Read the model definition and answer for the solid it produces. Units are mm, in the model's axes. A direction names the side the tool comes from. Coordinates: 2 decimals unless noted, no trailing zeros. Loops run counter-clockwise (first coordinate to the right, second up) from the corner with the lowest first, then second, coordinate; pieces in that order, holes last. Notation, with made-up numbers: M 13.25,31 L 17.25,31 A8 cw 17.25,35 Z; hole C 10.25,-10.75 d3. An arc over 180 degrees is marked long. One line per item, written item: value. Start each with the question number.
```python
from build123d import *

# Parameters (mm, degrees)
SKETCH1_R            = 1.5
SKETCH1_R_2          = 2.5
BOSS_EXTRUDE1_DEPTH  = 5
M2_CLEARANCE_HOLE1_D = 2.4
FILLET1_R            = 2
BOSS_EXTRUDE2_START  = 5
BOSS_EXTRUDE2_DEPTH  = 5
CUT_EXTRUDE1_START   = -3
SKETCH5_R            = 1.5
CUT_EXTRUDE1_DEPTH   = 3
CUT_EXTRUDE2_START   = -2
SKETCH6_R            = 1.2
CUT_EXTRUDE2_DEPTH   = 2


with BuildPart() as part:
    # Sketch1 → Boss-Extrude1 (new body)
    # profile 1 of 3: a face of its own
    with BuildSketch(Plane(origin=(0, 0, 0), x_dir=(1, 0, 0), z_dir=(0, 1, 0))):
        with BuildLine():
            Line((10.5, 2.5), (-10.5, 2.5))
            ThreePointArc((-10.5, 2.5), (-8.732233047, 1.767766953), (-8, 0))
            ThreePointArc((-8, 0), (-10.997961344, -2.449904998), (-12.8016276, 0.975966388))
            Line((-12.8016276, 0.975966388), (-18.090408136, -11.496597633))
            Line((-18.090408136, -11.496597633), (-13.587005769, -16))
            Line((-13.587005769, -16), (13.587005769, -16))
            Line((13.587005769, -16), (18.090408136, -11.496597633))
            Line((18.090408136, -11.496597633), (12.8016276, 0.975966388))
            ThreePointArc((12.8016276, 0.975966388), (12.949904998, 0.497961344), (13, 0))
            ThreePointArc((13, 0), (8.732233047, -1.767766953), (10.5, 2.5))
        make_face()
        with Locations(Location((-14.4, -12.5, 0), (0, 0, 270))):
            Circle(SKETCH1_R, mode=Mode.SUBTRACT)
        with Locations(Location((14.4, -12.5, 0), (0, 0, 270))):
            Circle(SKETCH1_R, mode=Mode.SUBTRACT)
        Polygon((-7.5, -12.5), (0, -2), (7.5, -12.5), align=None, mode=Mode.SUBTRACT)
    # profile 2 of 3: a face of its own
    with BuildSketch(Plane(origin=(0, 0, 0), x_dir=(1, 0, 0), z_dir=(0, 1, 0))):
        with Locations((-10.5, 0)):
            Circle(SKETCH1_R_2)
    # profile 3 of 3: a face of its own
    with BuildSketch(Plane(origin=(0, 0, 0), x_dir=(1, 0, 0), z_dir=(0, 1, 0))):
        with Locations((10.5, 0)):
            Circle(SKETCH1_R_2)
    extrude(amount=BOSS_EXTRUDE1_DEPTH)

    # M2 Clearance Hole1 (through all)
    with Locations(Plane(origin=(0, 5, 0), x_dir=(1, 0, 0), z_dir=(0, 1, 0))):
        with Locations((-10.5, 0), (10.5, 0)):
            Hole(M2_CLEARANCE_HOLE1_D / 2)

    # Fillet1
    fillet1_edges = [part.edges().sort_by_distance(p)[0] for p in [
        (0, 2.5, 2),
        (-7.5, 2.5, 12.5),
        (7.5, 2.5, 12.5),
    ]]
    fillet(fillet1_edges, radius=FILLET1_R)

    # Sketch4 → Boss-Extrude2 (add)
    with BuildSketch(Plane.XZ.offset(BOSS_EXTRUDE2_START)):
        with BuildLine():
            Line((-14.101857368, 15.4851484), (-17.3851484, 12.201857368))
            ThreePointArc((-17.3851484, 12.201857368), (-15.317017203, 9.643589762), (-12.146233974, 10.519964975))
            ThreePointArc((-12.146233974, 10.519964975), (-12.695571974, 11.154604627), (-13.01161859, 11.932199807))
            ThreePointArc((-13.01161859, 11.932199807), (-15.9, 12.5), (-13.01161859, 13.067800193))
            ThreePointArc((-13.01161859, 13.067800193), (-12.695571974, 13.845395373), (-12.146233974, 14.480035025))
            ThreePointArc((-12.146233974, 14.480035025), (-13.028642033, 15.168216132), (-14.101857368, 15.4851484))
        make_face()
        with BuildLine():
            ThreePointArc((12.146233974, 10.519964975), (15.317017203, 9.643589762), (17.3851484, 12.201857368))
            Line((17.3851484, 12.201857368), (14.101857368, 15.4851484))
            ThreePointArc((14.101857368, 15.4851484), (13.028642033, 15.168216132), (12.146233974, 14.480035025))
            ThreePointArc((12.146233974, 14.480035025), (12.695571974, 13.845395373), (13.01161859, 13.067800193))
            ThreePointArc((13.01161859, 13.067800193), (15.9, 12.5), (13.01161859, 11.932199807))
            ThreePointArc((13.01161859, 11.932199807), (12.695571974, 11.154604627), (12.146233974, 10.519964975))
        make_face()
    extrude(amount=-BOSS_EXTRUDE2_DEPTH)

    # Sketch5 → Cut-Extrude1 (cut)
    # profile 1 of 2: a face of its own
    with BuildSketch(Plane(origin=(0, 5, 0), x_dir=(1, 0, 0), z_dir=(0, 1, 0)).offset(CUT_EXTRUDE1_START)):
        Polygon((15.109788915, -15.148968295), (17.048968295, -13.209788915), (16.33917938, -10.56082062), (13.690211085, -9.851031705), (11.751031705, -11.790211085), (12.46082062, -14.43917938), align=None)
        with Locations(Location((14.4, -12.5, 0), (0, 0, 157.757128517))):
            Circle(SKETCH5_R, mode=Mode.SUBTRACT)
    # profile 2 of 2: a face of its own
    with BuildSketch(Plane(origin=(0, 5, 0), x_dir=(1, 0, 0), z_dir=(0, 1, 0)).offset(CUT_EXTRUDE1_START)):
        Polygon((-12.46082062, -14.43917938), (-15.109788915, -15.148968295), (-17.048968295, -13.209788915), (-16.33917938, -10.56082062), (-13.690211085, -9.851031705), (-11.751031705, -11.790211085), align=None)
    extrude(amount=CUT_EXTRUDE1_DEPTH, mode=Mode.SUBTRACT)

    # Sketch6 → Cut-Extrude2 (cut)
    # profile 1 of 6: a face of its own
    with BuildSketch(Plane(origin=(0, 5, 0), x_dir=(1, 0, 0), z_dir=(0, 1, 0)).offset(CUT_EXTRUDE2_START)):
        with BuildLine():
            Line((-7.757586221, 0), (-9.128793111, 2.375))
            Line((-9.128793111, 2.375), (-11.28062475, 2.375))
            ThreePointArc((-11.28062475, 2.375), (-11.75, 2.165063509), (-12.166497959, 1.863540864))
            Line((-12.166497959, 1.863540864), (-13.140949749, 0.175740855))
            Line((-13.140949749, 0.175740855), (-13.226879096, -0.026906859))
            Line((-13.226879096, -0.026906859), (-11.871206889, -2.375))
            Line((-11.871206889, -2.375), (-9.128793111, -2.375))
            Line((-9.128793111, -2.375), (-7.757586221, 0))
        make_face()
        with Locations(Location((-10.5, 0, 0), (0, 0, 270))):
            Circle(SKETCH6_R, mode=Mode.SUBTRACT)
    # profile 2 of 6: a face of its own
    with BuildSketch(Plane(origin=(0, 5, 0), x_dir=(1, 0, 0), z_dir=(0, 1, 0)).offset(CUT_EXTRUDE2_START)):
        with BuildLine():
            Line((-13.140949749, 0.175740855), (-12.166497959, 1.863540864))
            ThreePointArc((-12.166497959, 1.863540864), (-12.533089331, 1.454835995), (-12.8016276, 0.975966388))
            Line((-12.8016276, 0.975966388), (-13.140949749, 0.175740855))
        make_face()
    # profile 3 of 6: a face of its own
    with BuildSketch(Plane(origin=(0, 5, 0), x_dir=(1, 0, 0), z_dir=(0, 1, 0)).offset(CUT_EXTRUDE2_START)):
        with BuildLine():
            Line((-9.128793111, 2.375), (-9.200961894, 2.5))
            Line((-9.200961894, 2.5), (-10.5, 2.5))
            ThreePointArc((-10.5, 2.5), (-10.895284708, 2.468552207), (-11.28062475, 2.375))
            Line((-11.28062475, 2.375), (-9.128793111, 2.375))
        make_face()
    # profile 4 of 6: a face of its own
    with BuildSketch(Plane(origin=(0, 5, 0), x_dir=(1, 0, 0), z_dir=(0, 1, 0)).offset(CUT_EXTRUDE2_START)):
        with BuildLine():
            Line((7.757586221, 0), (9.128793111, -2.375))
            Line((9.128793111, -2.375), (11.871206889, -2.375))
            Line((11.871206889, -2.375), (13.226879096, -0.026906859))
            Line((13.226879096, -0.026906859), (13.140949749, 0.175740855))
            Line((13.140949749, 0.175740855), (12.166497959, 1.863540864))
            ThreePointArc((12.166497959, 1.863540864), (11.75, 2.165063509), (11.28062475, 2.375))
            Line((11.28062475, 2.375), (9.128793111, 2.375))
            Line((9.128793111, 2.375), (7.757586221, 0))
        make_face()
        with Locations(Location((10.5, 0, 0), (0, 0, 270))):
            Circle(SKETCH6_R, mode=Mode.SUBTRACT)
    # profile 5 of 6: a face of its own
    with BuildSketch(Plane(origin=(0, 5, 0), x_dir=(1, 0, 0), z_dir=(0, 1, 0)).offset(CUT_EXTRUDE2_START)):
        with BuildLine():
            Line((12.166497959, 1.863540864), (13.140949749, 0.175740855))
            Line((13.140949749, 0.175740855), (12.8016276, 0.975966388))
            ThreePointArc((12.8016276, 0.975966388), (12.533089331, 1.454835995), (12.166497959, 1.863540864))
        make_face()
    # profile 6 of 6: a face of its own
    with BuildSketch(Plane(origin=(0, 5, 0), x_dir=(1, 0, 0), z_dir=(0, 1, 0)).offset(CUT_EXTRUDE2_START)):
        with BuildLine():
            Line((9.200961894, 2.5), (9.128793111, 2.375))
            Line((9.128793111, 2.375), (11.28062475, 2.375))
            ThreePointArc((11.28062475, 2.375), (10.895284708, 2.468552207), (10.5, 2.5))
            Line((10.5, 2.5), (9.200961894, 2.5))
        make_face()
    extrude(amount=CUT_EXTRUDE2_DEPTH, mode=Mode.SUBTRACT)


solid = part.part
```
1) A tool of negligible diameter and unlimited length cuts with its end or side. For faces 4 (the face through (3.409, 2.465, 6.773)), 5 (the face through (12.7, -2.54, 11.16)), 6 (the face through (-15.363, -2.535, 9.659)), from which of +Z, -Z, +X, -X, +Y, -Y can it reach the whole face along a straight path? Write none if from no direction.
2) Section A-A (y = 2.5) is taken. Determine the outline of the cut face in (x, z), then the cut area to 3 significant figures.
3) Section C-C (y = -1.5) is taken. Determine the outline of the cut face in (x, z) (3 decimals), then the cut area to 3 significant figures.
4) Section D-D (z = 6.75) is taken. Determine the outline of the cut face in (x, y), then the cut area to 3 significant figures.
5) Flat-ended cylindrical pins translate along their axes: pin 1 (4 mm diameter, centred on x = 10.5, z = 1, fed in from +Y); pin 2 (1.5 mm diameter, centred on x = -13, z = 12, fed in from +Y); pin 3 (3 mm diameter, centred on x = 10.5, z = 0, fed in from +Y); pin 4 (1 mm diameter, centred on y = 3.5, z = 0, fed in from -X). Find the tip coordinate at first contact, or state that the pin passes through.
6) Section B-B (x = 3) is taken. Determine the outline of the cut face in (y, z).
7) Consider line 1 along Z through (x, y) = (10.5, 1.5); line 2 along X through (y, z) = (2.5, -1); line 3 along X through (y, z) = (1.45, 0). Determine where each line is inside the solid, lowest interval first.
8) For a pull along X with two mould halves and no side action, classify faces 1 (the face through (-16.63, 3.48, 11.64)), 2 (the face through (13.51, 3.48, 14.72)), 3 (the face through (-15.807, -0.07, 13.78)) as released by +X, released by -X, zero draft, split by the parting line, or undercut.
Results found:
1. face 4: +Y, -Y
1. face 5: -Y
1. face 6: -Z, -Y
2. outline: M -18.09,11.5 L -12.8,-0.98 A2.5 ccw -10.5,-2.5 L 10.5,-2.5 A2.5 ccw 12.8,-0.98 L 18.09,11.5 L 16.91,12.68 L 16.34,10.56 L 13.69,9.85 L 11.75,11.79 L 12.46,14.44 L 14.58,15.01 L 13.59,16 L -13.59,16 L -14.58,15.01 L -12.46,14.44 L -11.75,11.79 L -13.69,9.85 L -16.34,10.56 L -16.91,12.68 Z; hole C -10.5,0 d2.4; hole M -5.24,9.34 L -1.63,4.28 A2 ccw 1.63,4.28 L 5.24,9.34 A2 ccw 3.61,12.5 L -3.61,12.5 A2 ccw Z; hole C 10.5,0 d2.4
2. area: 450 mm²
3. outline: M -17.385,12.202 A3 ccw -12.146,10.52 A2.575 cw -13.012,11.932 A1.5 cw long -13.012,13.068 A2.575 cw -12.146,14.48 A3 ccw -14.102,15.485 Z; M 12.146,10.52 A3 ccw 17.385,12.202 L 14.102,15.485 A3 ccw 12.146,14.48 A2.575 cw 13.012,13.068 A1.5 cw long 13.012,11.932 A2.575 cw Z
3. area: 26.4 mm²
4. outline: M -16.08,0 L -3.39,0 L -3.39,5 L -16.08,5 Z; M 3.39,0 L 16.08,0 L 16.08,5 L 3.39,5 Z
4. area: 127 mm²
5. pin 1: stops at y = 5
5. pin 2: stops at y = 2
5. pin 3: stops at y = 3
5. pin 4: stops at x = -13.43
6. outline: M 0,-2.5 L 5,-2.5 L 5,6.2 L 0,6.2 Z; M 0,12.5 L 5,12.5 L 5,16 L 0,16 Z
7. line 1: z = -2.5 to -1.2, 1.2 to 16
7. line 2: x = -12.79 to -11.16, -9.84 to 9.84, 11.16 to 12.79
7. line 3: x = -13.22 to -11.7, -9.3 to 9.3, 11.7 to 13.22
8. face 1: undercut
8. face 2: released by +X
8. face 3: released by -X
